Design review of the part built by this model. Coordinates are the model's own, in mm. Give positions to 0.01 mm unless a question says otherwise; leave off trailing zeros. Write each loop counter-clockwise with the first axis right and the second up, starting at its lowest first coordinate (ties: lowest second). Pieces come first, ordered by that corner, then holes.
```python
from build123d import *

# Parameters (mm, degrees)
F1_DEPTH = 914.4
F2_R     = 9.525
F3_DEPTH = 41.8348
F5_DEPTH = 41.8348
F6_R     = 5.55625
F7_DEPTH = 41.8348


with BuildPart() as f1:
    # F0 (on Top) → F1 (new body)
    with BuildSketch(Plane.XY):
        with BuildLine():
            Line((-50.8, 41.8338), (-50.8, 0))
            Line((-50.8, 0), (50.8, 0))
            Line((50.8, 0), (50.8, 41.8338))
            ThreePointArc((50.8, 41.8338), (48.9940285402, 41.1716778311), (48.0440153768, 39.4991307706))
            Line((48.0440153768, 39.4991307706), (43.4969259811, 12.216594402))
            ThreePointArc((43.4969259811, 12.216594402), (41.078710656, 7.9592018846), (36.4816923948, 6.2738))
            Line((36.4816923948, 6.2738), (-36.4816923948, 6.2738))
            ThreePointArc((-36.4816923948, 6.2738), (-41.078710656, 7.9592018846), (-43.4969259811, 12.216594402))
            Line((-43.4969259811, 12.216594402), (-48.0440153768, 39.4991307706))
            ThreePointArc((-48.0440153768, 39.4991307706), (-48.9940285402, 41.1716778311), (-50.8, 41.8338))
        make_face()
    extrude(amount=F1_DEPTH)

    # F2 (on face) → F3 (cut, through all)
    with BuildSketch(Plane.XZ):
        with Locations((0, 38.1)):
            Circle(F2_R)
    extrude(amount=-F3_DEPTH, mode=Mode.SUBTRACT)

    # F4 (on face) → F5 (cut, through all)
    with BuildSketch(Plane.XZ):
        with BuildLine():
            Line((8.73125, 867.0375161499), (8.73125, 876.3))
            ThreePointArc((8.73125, 876.3), (0, 885.03125), (-8.73125, 876.3))
            Line((-8.73125, 876.3), (-8.73125, 867.0375161499))
            ThreePointArc((-8.73125, 867.0375161499), (0, 831.05625), (8.73125, 867.0375161499))
        make_face()
    extrude(amount=-F5_DEPTH, mode=Mode.SUBTRACT)

    # F6 (on face) → F7 (cut, through all)
    with BuildSketch(Plane.XZ):
        with Locations((-22.225, 714.0829)):
            Circle(F6_R)
        with Locations((22.225, 714.0829)):
            Circle(F6_R)
        with Locations((-22.225, 234.6579)):
            Circle(F6_R)
        with Locations((22.225, 234.6579)):
            Circle(F6_R)
    extrude(amount=-F7_DEPTH, mode=Mode.SUBTRACT)


solid = f1.part
```
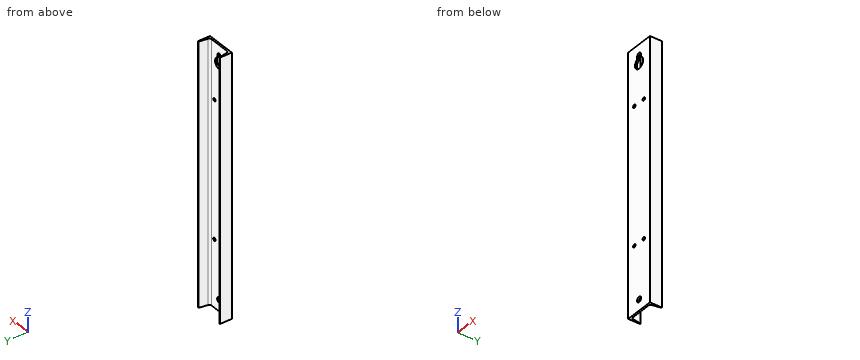
(1) Clearance check with flat-ended pins moving along their axes: P1, Ø12, axis at x = -19.5, z = 610, coming from the +Y side; P2, Ø18, axis at x = -22.22, z = 714.08, coming from the -Y side. State where each tip first meets the part, or that it passes through.
Resolved:
P1: stops at y = 6.27
P2: stops at y = 0
(2) To check wall thickness, follow L1, parallel to Z at x = 0, y = 2 (3 decimals); L2, parallel to Y at x = 32, z = 642; L3, parallel to X at y = 23, z = 209. State the ranges of each line that lie inside material, in increasing order.
Resolved:
L1: z = 0 to 28.575, 47.625 to 831.056, 885.031 to 914.4
L2: y = 0 to 6.27
L3: x = -50.8 to -45.29, 45.29 to 50.8
(3) Consider section B-B, the plane x = 0. Give the boundary of the cut face in (y, z) (3 decimals), then the cut area to 3 significant figures.
Resolved:
outline: (0, 0) - (6.274, 0) - (6.274, 28.575) - (0, 28.575) - close; (0, 47.625) - (6.274, 47.625) - (6.274, 831.056) - (0, 831.056) - close; (0, 885.031) - (6.274, 885.031) - (6.274, 914.4) - (0, 914.4) - close
area: 5,280 mm2
(4) Consider section C-C, the plane y = 27. Give the boundary of the cut face in (x, z), then the cut area to 3 significant figures.
Resolved:
outline: (-50.8, 0) - (-45.96, 0) - (-45.96, 914.4) - (-50.8, 914.4) - close; (45.96, 0) - (50.8, 0) - (50.8, 914.4) - (45.96, 914.4) - close
area: 8,850 mm2
(5) Consider section A-A, the plane z = 38.1. Give the boundary of the cut face in (x, y) (3 decimals), then the cut area to 3 significant figures.
Resolved:
outline: (-50.8, 0) - (-9.525, 0) - (-9.525, 6.274) - (-36.482, 6.274) arc R7.112 cw to (-43.497, 12.217) - (-48.044, 39.499) arc R2.794 ccw to (-50.8, 41.834) - close; (9.525, 0) - (50.8, 0) - (50.8, 41.834) arc R2.794 ccw to (48.044, 39.499) - (43.497, 12.217) arc R7.112 cw to (36.482, 6.274) - (9.525, 6.274) - close
area: 909 mm2
